Read the model definition and answer for the solid it produces. Units are mm, in the model's axes. Face numbers are marked on the shaded views. A direction names the side the tool comes from. Give positions to 0.01 mm unless a question says otherwise; leave off trailing zeros. Loops run counter-clockwise (first coordinate to the right, second up) from the corner with the lowest first, then second, coordinate; pieces in that order, holes last. Notation, with made-up numbers: (-24.5, 83) - (-14.5, 83) arc R37 ccw to (-14.5, 121) - close; hole circle Ø4 at (-4, 32). An arc over 180 degrees is marked (long way). Put each result on its own line as item: value. Start each with the question number.
1. Given pin 1 Ø9 at (x, y) = (65, 0) entering from +Z; pin 2 Ø5.5 at (x, y) = (15, 0) entering from -Z; pin 3 Ø1 at (y, z) = (9.5, 2) entering from -X; pin 4 Ø1.5 at (y, z) = (9, 4) entering from -X, each flat-ended and moving along its own axis, determine where each tip first touches the part or whether it passes through.
2. A cutting plane is placed at D-D, the plane z = 2.45. Determine the outline of the cut face in (x, y), plus the area to 3 significant figures.
3. A cutting plane is placed at A-A, the plane x = 45. Determine the outline of the cut face in (y, z).
4. A cutting plane is placed at C-C, the plane y = -1. Determine the outline of the cut face in (x, z).
5. For a pull along Y with two mould halves and no side action, classify the marked faces 1, 2 and 3 as released by +Y, released by -Y, zero draft, split by the parting line, or undercut.
6. A cutting plane is placed at B-B, the plane z = 5.3. Determine the outline of the cut face in (x, y), plus the area to 3 significant figures.
7. For the marked faces 4 and 5, determine the directions among +Z, -Z, +X, -X, +Y, -Y from which every point of the face is accessible in a straight line to the end or side of a thin tool.
8. Consider L1, parallel to Y at x = 65, z = 4.4; L2, parallel to Y at x = 15, z = 0.75; L3, parallel to X at y = 1, z = 0.85. Determine where each line is inside the solid, lowest interval first. Write a range as from..to.
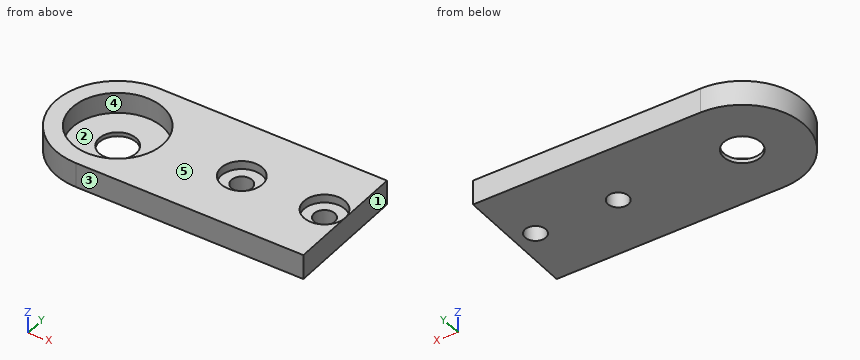
Autodesk Inventor part; units mm, degrees
ref_plane "YZ Plane" through (0, 0, 0) normal (1, 0, 0) x (0, 1, 0)
ref_plane "XZ Plane" through (0, 0, 0) normal (0, 1, 0) x (-1, 0, 0)
ref_plane "XY Plane" through (0, 0, 0) normal (0, 0, 1) x (1, 0, 0)
sketch "Sketch1" plane through (0, 0, 0) normal (0, 0, 1) x (1, 0, 0)
  line L0 (15, 15) -> (70, 15)
  line L1 (70, 15) -> (70, -15)
  line L2 (70, -15) -> (15, -15)
  line L3 (-14, 0) -> (84, 0)
  arc A0 (15, 15) -> (15, -15) centre (15, 0) ccw
  line L4 (0, -21) -> (0, 21)
  line L5 (15, 0) -> (70, 0)
  point P0 (0, 0)
  dimension "d4" = 30
  dimension "d15" = 15
  dimension "d16" = 55
extrude "Extrusion1" add sketch "Sketch1" along normal blind 6
sketch "Sketch2" plane through (0, 0, 6) normal (0, 0, 1) x (1, 0, 0)
  circle A0 centre (15, 0) radius 11
  arc A1 (15, 15) -> (15, -15) centre (15, 0) ccw
  point P0 (0, 0)
  dimension "d7" = 22
extrude "Extrusion2" cut sketch "Sketch2" against normal blind 10
sketch "Sketch3" plane through (0, 0, 6) normal (0, 0, 1) x (1, 0, 0)
  circle A0 centre (65, 0) radius 2.5
  line L0 (70, -15) -> (70, 15)
  circle A1 centre (45, 0) radius 2.5
  point P0 (0, 0)
  dimension "d10" = 5
  dimension "d12" = 5
  dimension "d26" = 5
  dimension "d27" = 20
extrude "Extrusion3" cut sketch "Sketch3" against normal blind 10
sketch "Sketch4" plane through (0, 0, 0) normal (0, 0, -1) x (-1, 0, 0)
  circle A0 centre (-15, 0) radius 15
  arc A1 (-15, -15) -> (-15, 15) centre (-15, 0) ccw
  circle A2 centre (-15, 0) radius 11
  point P0 (0, 0)
extrude "Extrusion4" add sketch "Sketch4" against normal blind 1 contours A0 | A2
sketch "Sketch6" plane through (0, 0, 6) normal (0, 0, 1) x (1, 0, 0)
  circle A0 centre (65, 0) radius 2.5
  circle A1 centre (65, 0) radius 5
  circle A2 centre (45, 0) radius 5
  circle A3 centre (45, 0) radius 2.5
  point P0 (0, 0)
  dimension "d22" = 10
  dimension "d28" = 10
extrude "Extrusion6" cut sketch "Sketch6" against normal blind 2
sketch "Sketch7" plane through (0, 0, 0) normal (0, 0, -1) x (-1, 0, 0)
  arc A0 (-15, -15) -> (-15, 15) centre (-15, 0) ccw
  circle A1 centre (-15, 0) radius 4.5
  point P0 (0, 0)
  dimension "d29" = 9
extrude "Extrusion7" cut sketch "Sketch7" against normal blind 2
properties part number "bearing_mount"
Return value:
1. pin 1: stops at z = 4
1. pin 2: passes through
1. pin 3: stops at x = 3
1. pin 4: stops at x = 2.47
2. outline: (15, -15) - (70, -15) - (70, 15) - (15, 15) arc R15 ccw to start; hole circle Ø22 at (15, 0); hole circle Ø5 at (45, 0); hole circle Ø5 at (65, 0)
2. area: 1,580 mm2
3. outline: (-15, 0) - (-2.5, 0) - (-2.5, 4) - (-5, 4) - (-5, 6) - (-15, 6) - close; (2.5, 0) - (15, 0) - (15, 6) - (5, 6) - (5, 4) - (2.5, 4) - close
4. outline: (0.03, 0) - (10.61, 0) - (10.61, 1) - (4.05, 1) - (4.05, 6) - (0.03, 6) - close; (19.39, 0) - (42.71, 0) - (42.71, 4) - (40.1, 4) - (40.1, 6) - (25.95, 6) - (25.95, 1) - (19.39, 1) - close; (47.29, 0) - (62.71, 0) - (62.71, 4) - (60.1, 4) - (60.1, 6) - (49.9, 6) - (49.9, 4) - (47.29, 4) - close; (67.29, 0) - (70, 0) - (70, 6) - (69.9, 6) - (69.9, 4) - (67.29, 4) - close
5. face 1: zero draft
5. face 2: undercut
5. face 3: released by -Y
6. outline: (15, -15) - (70, -15) - (70, 15) - (15, 15) arc R15 ccw to start; hole circle Ø22 at (15, 0); hole circle Ø10 at (45, 0); hole circle Ø10 at (65, 0)
6. area: 1,470 mm2
7. face 4: +Z
7. face 5: +Z, +X, -X, +Y, -Y
8. L1: y = -15..-5, 5..15
8. L2: y = -15..-4.5, 4.5..15
8. L3: x = 0.03..10.61, 19.39..42.71, 47.29..62.71, 67.29..70
